The model under review builds one solid part; all positions refer to its coordinate system, in mm. A direction names the side the tool comes from. Give positions to 0.01 mm unless a question says otherwise; leave off trailing zeros. Order: outer loops, then holes, each group sorted by start corner. A loop starts at its lowest first (then second) coordinate and runs counter-clockwise, first axis right, second up. Notation, with made-up numbers: (81.25, 7.5) - (107.25, 7.5) arc R30 ccw to (107.25, 35.5) - close; hole circle Ø6 at (-22, 46.25). An arc over 180 degrees is marked (long way). Put each result on its own line as item: value.
```python
from build123d import *

# Parameters (mm, degrees)
CYLINDER002_R         = 4
CYLINDER002_DEPTH     = 3
CYLINDER001_R         = 4
CYLINDER001_DEPTH     = 3
TORUS_R               = 2
TORUS_ANGLE           = 120
TORUS_PLACEMENT_ANGLE = 60
CYLINDER_R            = 25
CYLINDER_DEPTH        = 3


with BuildPart() as cilindre002:
    # Cylinder002 → Cylinder002 (new body)
    with BuildSketch(Plane(origin=(-10, -9, 1), x_dir=(1, 0, 0), z_dir=(0, 0, 1))):
        Circle(CYLINDER002_R)
    extrude(amount=CYLINDER002_DEPTH)


with BuildPart() as fusion:
    # Cylinder001 → Cylinder001 (new body)
    with BuildSketch(Plane(origin=(-10, 9, 1), x_dir=(1, 0, 0), z_dir=(0, 0, 1))):
        Circle(CYLINDER001_R)
    extrude(amount=CYLINDER001_DEPTH)

    # Fusion: union Cilindre002
    add(cilindre002.part)


with BuildPart() as torus:
    # Torus → Torus (revolve)
    with BuildSketch(Plane.XZ):
        with Locations((13, 0)):
            Circle(TORUS_R)
    revolve(axis=Axis((0, 0, 0), (0, 0, 1)), revolution_arc=TORUS_ANGLE)


with BuildPart() as torus_1:
    # Torus placement: moved
    add(torus.part.moved(Location((0, 0, 3))).rotate(Axis((0, 0, 3), (0, 0, -1)), TORUS_PLACEMENT_ANGLE))


with BuildPart() as cut001:
    # Cylinder → Cylinder (new body)
    with BuildSketch(Plane.XY):
        Circle(CYLINDER_R)
    extrude(amount=CYLINDER_DEPTH)

    # Cut: cut Torus
    add(torus_1.part, mode=Mode.SUBTRACT)

    # Cut001: cut Fusion
    add(fusion.part, mode=Mode.SUBTRACT)


solid = cut001.part
```
(1) Take a section at D-D, the plane y = 14. Write out the cut boundary in (x, z), then the cut area to 3 significant figures.
The answers:
outline: (-20.71, 0) - (20.71, 0) - (20.71, 3) - (-20.71, 3) - close
area: 124 mm^2
(2) Clearance check with flat-ended pins moving along their axes: pin 1 Ø1 at (y, z) = (-19.5, 1.5) entering from +X; pin 2 Ø1 at (x, z) = (-1, 2.5) entering from -Y (3 decimals); pin 3 Ø6.5 at (x, y) = (-10, -9) entering from +Z. State where each tip first meets the part, or that it passes through.
The answers:
pin 1: x = 16.25
pin 2: y = -24.995
pin 3: z = 1
(3) Wall thickness on L1, parallel to Y at x = -10, z = 2.65; L2, parallel to X at y = 9, z = 2.6; L3, parallel to X at y = -9, z = 1.7: over which ranges is each line inside the solid? List them lowest first.
The answers:
L1: -22.91 to -13, -5 to 5, 13 to 22.91
L2: -23.32 to -14, -6 to 6.39, 11.95 to 23.32
L3: -23.32 to -14, -6 to 7.13, 11.39 to 23.32
(4) The part is to be moulded in two halves that separate along X. For faces 3 (the cylindrical face through (23.846, 7.509, 1.479)), 4 (the flat face through (0, 0, 3)), 5 (the flat face through (-10, 9, 1)), say which applies: pulls with the +X half, pulls with the -X half, needs draft (parallel to the pull), parting line crosses it, or undercut.
The answers:
face 3: parting line crosses it
face 4: needs draft
face 5: undercut
(5) For faces 1 (the flat face through (0, 0, 0)), 2 (the flat face through (6.486, 11.234, 2.236)), list the 3-axis set-ups (+Z, -Z, +X, -X, +Y, -Y) from which the entire face can be reached by the end or side of a thin tool; tool diameter is ignored.
The answers:
face 1: -Z, +X, -X, +Y, -Y
face 2: +Z
(6) Take a section at C-C, the plane x = -10. Write out the cut boundary in (y, z), then the cut area to 3 significant figures.
The answers:
outline: (-22.91, 0) - (22.91, 0) - (22.91, 3) - (13, 3) - (13, 1) - (5, 1) - (5, 3) - (-5, 3) - (-5, 1) - (-13, 1) - (-13, 3) - (-22.91, 3) - close
area: 105 mm^2
(7) Take a section at B-B, the plane y = 0. Write out the cut boundary in (x, z), then the cut area to 3 significant figures.
The answers:
outline: (-25, 0) - (25, 0) - (25, 3) - (15, 3) arc R2 cw to (11, 3) - (-25, 3) - close
area: 144 mm^2
(8) Take a section at A-A, the plane z = 2.4. Write out the cut boundary in (x, y), then the cut area to 3 significant figures.
The answers:
outline: circle Ø50 at (0, 0); hole circle Ø8 at (-10, -9); hole circle Ø8 at (-10, 9); hole (5.55, -9.61) - (7.45, -12.91) arc R14.91 ccw to (7.45, 12.91) - (5.55, 9.61) arc R11.09 cw to start
area: 1,760 mm^2
